Build history of the part. All positions in model axes, mm. Face numbers are marked on the shaded views. Coordinates: 2 decimals unless noted, no trailing zeros. Write each loop counter-clockwise with the first axis right and the second up, starting at its lowest first coordinate (ties: lowest second). Pieces come first, ordered by that corner, then holes. Notation, with made-up numbers: (82, -21.75) -> (92, -21.75) arc R14 cw to (92, -2.75) -> close; hole circle Ø3 at (-21, -17.75). An arc over 180 degrees is marked (long way). Write each question's results on one line, items separated by ' | '. Start each with the question number.
Q1. Drill centre lines: line 1 (Y direction, x = -2, z = 34); line 2 (Z direction, x = -18, y = 87); line 3 (X direction, y = 160.5, z = 18.5). Where is each one in solid material? Low to high.
Q2. Saw through at A-A on x = 0. Give the cut face in (y, z).
Q3. Saw through at C-C on z = 11.5. Give the cut face in (x, y), and give its area (3 significant figures).
Q4. Drop flat-ended pins along their axis: pin 1 Ø6 at (y, z) = (112.5, 20) entering from -X; pin 2 Ø1.5 at (y, z) = (72, 11) entering from +X; pin 3 Ø8 at (x, y) = (1, 101.5) entering from -Z. Give the stop position or say it passes through.
Q5. Saw through at B-B on y = 89. Give the cut face in (x, z).
Q6. Two-plate mould, pull along Y, no slides. Class the marked faces 1, 2 and 3: released by +Y, released by -Y, zero draft, split by the parting line, or undercut.
Solid Edge part; units mm, degrees
sketch "Sketch1" plane through (0, 0, 0) normal (0, -1, 0) x (1, 0, 0)
  circle A0 centre (0, 0) radius 30
extrude "Protrusion1" add sketch "Sketch1" against normal blind 170
sketch "Sketch2" plane through (0, 0, 0) normal (0, -1, 0) x (1, 0, 0)
  circle A0 centre (0, 0) radius 45
extrude "ExtrudedProtrusion_2" add sketch "Sketch2" against normal blind 10
mirror "Mirror1" about plane through (0, 85, 0) normal (0, -1, 0) of "ExtrudedProtrusion_2"
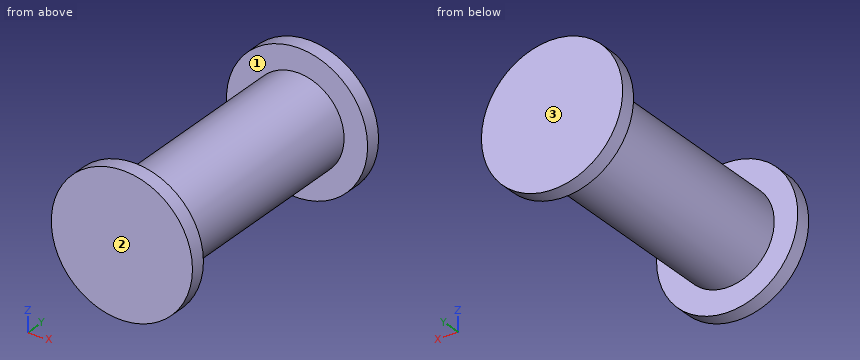
Returned:
1) line 1: y = 0 to 10, 160 to 170 | line 2: z = -24 to 24 | line 3: x = -41.02 to 41.02
2) outline: (0, -45) -> (10, -45) -> (10, -30) -> (160, -30) -> (160, -45) -> (170, -45) -> (170, 45) -> (160, 45) -> (160, 30) -> (10, 30) -> (10, 45) -> (0, 45) -> close
3) outline: (-43.51, 0) -> (43.51, 0) -> (43.51, 10) -> (27.71, 10) -> (27.71, 160) -> (43.51, 160) -> (43.51, 170) -> (-43.51, 170) -> (-43.51, 160) -> (-27.71, 160) -> (-27.71, 10) -> (-43.51, 10) -> close | area: 10,100 mm2
4) pin 1: stops at x = -24.72 | pin 2: stops at x = 28.19 | pin 3: stops at z = -30
5) outline: circle Ø60 at (0, 0)
6) face 1: undercut | face 2: released by -Y | face 3: released by +Y
